Here's how the part is built. I have some questions about the finished solid (model axes, mm). Round coordinates to 2 decimals unless told otherwise and drop trailing zeros. Answer as a JSON object with one key per item and string values. Group by question number.
1) I want a section at A-A, the plane z = 3.25. Give the number of separate pieces and of enclosed holes in the cut face, then the cut area to 3 significant figures.
2) Will these pins go through, and if not, where does the flat tip stop? P1, Ø0.8, axis at y = 1, z = 16.5, coming from the -X side; P2, Ø3.5, axis at y = -41, z = 2, coming from the +X side; P3, Ø1.7, axis at y = 24.5, z = 16.5, coming from the +X side (3 decimals).
3) If I drill on line 1 along Y through (x, z) = (50, 5); line 2 along X through (y, z) = (56, 12.25) (1 decimal); line 3 along X through (y, z) = (-42, 1.75), over which ranges is the centre line in solid material (lowest first)? Write a range as [from, to].
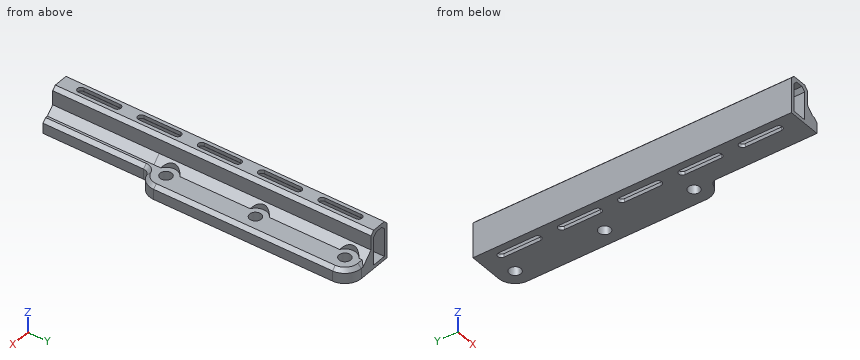
Autodesk Inventor part; units mm, degrees
ref_plane "Work Plane1" through (0, 0, 0) normal (0, 0, 1) x (1, 0, 0)
ref_plane "Work Plane2" through (40.2375, 90.7678, 31.75) normal (0, 0, 1) x (1, 0, 0)
ref_plane "Work Plane3" through (-55.775, -68.275, 0) normal (0, 0, 1) x (1, 0, 0)
ref_plane "Work Plane1" through (0, 0, 0) normal (0, 0, 1) x (1, 0, 0)
sketch "Sketch1" plane through (0, 0, 0) normal (0, 0, 1) x (1, 0, 0)
  circle A0 centre (50, -17.5) radius 2.6
  circle A1 centre (50, 22.5) radius 2.6
  circle A2 centre (50, 62.5) radius 2.6
  circle A3 centre (50, -17.5) radius 7.3625 construction
  circle A4 centre (50, 22.5) radius 7.3625 construction
  circle A5 centre (50, 62.5) radius 7.3625 construction
  line L0 (50, -24.8625) -> (42.6375, -24.8625)
  line L1 (42.6375, -24.8625) -> (42.6375, 69.8625)
  line L2 (42.6375, 69.8625) -> (50, 69.8625)
  line L3 (57.3625, -17.5) -> (57.3625, 62.5)
  arc A6 (50, -24.8625) -> (57.3625, -17.5) centre (50, -17.5) ccw
  arc A7 (57.3625, 62.5) -> (50, 69.8625) centre (50, 62.5) ccw
  circle A8 centre (50, -17.5) radius 5 construction
  point P0 (0, 0)
  dimension "d0" = 4.7625
  dimension "d1" = 10
extrude "Extrusion1" add sketch "Sketch1" along normal blind 6.175
sketch "Sketch2" plane through (0, 0, 6.175) normal (0, 0, 1) x (1, 0, 0)
  line L0 (42.6375, 69.8625) -> (42.6375, -24.8625)
  circle A0 centre (50, -17.5) radius 2.6
  circle A1 centre (50, -17.5) radius 5 construction
  line L1 (42.6375, -24.8625) -> (50, -24.8625) construction
  line L2 (44.225, -24.8625) -> (44.225, 69.8625)
  line L3 (42.6375, 69.8625) -> (44.225, 69.8625)
  line L4 (42.6375, -24.8625) -> (44.225, -24.8625)
  point P0 (0, 0)
  dimension "d4" = 10
  dimension "d34" = 1.5875
ref_plane "Work Plane2" through (40.2375, 90.7678, 31.75) normal (0, 0, 1) x (1, 0, 0)
extrude "Extrusion2" add sketch "Sketch2" along normal blind 9.525 contours L3 L2 L4 L0
chamfer "Chamfer1" distance 3.175 angle 45 1 edges at (44.225, 22.5, 6.175)
sketch "Sketch3" plane through (0, 0, 6.175) normal (0, 0, 1) x (1, 0, 0)
  circle A0 centre (50, -17.5) radius 2.6
  circle A1 centre (50, -17.5) radius 5
  circle A2 centre (50, 22.5) radius 2.6
  circle A3 centre (50, 62.5) radius 2.6
  circle A4 centre (50, 22.5) radius 5
  circle A5 centre (50, 62.5) radius 5
  point P0 (0, 0)
  point P1 (48.175, -15.6481)
  point P2 (48.175, -19.3519)
  point P3 (48.175, 24.3519)
  point P4 (48.175, 20.6481)
  point P5 (48.175, 64.3519)
  point P6 (48.175, 60.6481)
  dimension "d10" = 10
extrude "Extrusion3" cut sketch "Sketch3" along normal blind 25.4 contours A0 | A1 | A2 | A3 | A4 | A5
sketch "Sketch4" plane through (0, 0, 15.7) normal (0, 0, 1) x (1, 0, 0)
  line L0 (42.6375, -24.8625) -> (44.225, -24.8625)
  line L1 (44.225, -24.8625) -> (34.7, -24.8625)
  line L2 (34.7, -24.8625) -> (34.7, 69.8625)
  line L3 (34.7, 69.8625) -> (44.225, 69.8625)
  line L4 (44.225, 69.8625) -> (44.225, -24.8625)
  line L5 (44.225, 69.8625) -> (42.6375, 69.8625)
  line L6 (34.7, -24.8625) -> (36.2875, -24.8625)
  line L7 (36.2875, -24.8625) -> (36.2875, 69.8625)
  line L8 (36.2875, 69.8625) -> (34.7, 69.8625)
  line L9 (34.7, 69.8625) -> (34.7, -24.8625)
  line L10 (42.6375, 69.8625) -> (42.6375, -24.8625)
  point P0 (0, 0)
  dimension "d13" = 9.525
  dimension "d15" = 1.5875
  dimension "d16" = 1.5875
ref_plane "Work Plane3" through (-55.775, -68.275, 0) normal (0, 0, 1) x (1, 0, 0)
extrude "Extrusion4" add sketch "Sketch4" against normal up to surface (15.7 mm away) contours L1 L2 L3 L7
sketch "Sketch5" plane through (0, 0, 15.7) normal (0, 0, 1) x (1, 0, 0)
  line L0 (34.7, -24.8625) -> (34.7, 69.8625)
  line L1 (50, 69.8625) -> (42.6375, 69.8625)
  line L2 (34.7, -24.8625) -> (44.225, -24.8625)
  line L3 (44.225, -24.8625) -> (44.225, 69.8625)
  line L4 (44.225, 69.8625) -> (34.7, 69.8625)
  line L5 (34.7, 69.8625) -> (34.7, -24.8625)
  line L6 (44.225, -24.8625) -> (44.225, 69.8625)
  point P0 (0, 0)
extrude "Extrusion5" add sketch "Sketch5" along normal blind 1.5875
chamfer "Chamfer2" distance 1.5875 angle 45 4 edges at (44.225, 22.5, 17.2875) (34.7, 22.5, 17.2875) (36.2875, 22.5, 15.7) (42.6375, 22.5, 15.7)
sketch "Sketch7" plane through (42.6375, -24.8625, 0) normal (0, -1, 0) x (1, 0, 0)
  point P0 (-42.6375, 0)
sketch "Sketch8" plane through (42.6375, -24.8625, 0) normal (0, -1, 0) x (1, 0, 0)
  line L0 (-7.9375, 15.7) -> (-6.35, 17.2875)
  line L1 (-7.9375, 0) -> (-7.9375, 15.7)
  line L2 (-6.35, 0) -> (-7.9375, 0)
  line L3 (-6.35, 14.1125) -> (-6.35, 0)
  line L4 (-4.7625, 15.7) -> (-6.35, 14.1125)
  line L5 (-4.7625, 15.7) -> (-1.5875, 15.7)
  line L6 (0, 14.1125) -> (-1.5875, 15.7)
  line L7 (0, 0) -> (0, 14.1125)
  line L8 (0, 0) -> (7.3625, 0)
  line L9 (7.3625, 0) -> (7.3625, 6.175)
  line L10 (4.7625, 6.175) -> (7.3625, 6.175)
  line L11 (1.5875, 9.35) -> (4.7625, 6.175)
  line L12 (1.5875, 9.35) -> (1.5875, 15.7)
  line L13 (0, 17.2875) -> (1.5875, 15.7)
  line L14 (-6.35, 17.2875) -> (0, 17.2875)
  point P0 (-42.6375, 0)
ref_plane "Work Plane4" through (-290, -72.5, -10.037) normal (0, -1, 0) x (1, 0, 0)
extrude "Extrusion7" add sketch "Sketch8" along normal up to surface (47.6375 mm away)
fillet "Fillet1" radius 3.175 1 edges at (50, -24.8625, 3.0875)
sketch "Sketch9" plane through (0, 0, 17.2875) normal (0, 0, 1) x (1, 0, 0)
  line L0 (36.2875, 69.8625) -> (36.2875, -72.5)
  line L1 (42.6375, 69.8625) -> (42.6375, -72.5)
  line L2 (39.4625, -63.3595) -> (39.4625, -47.1256) construction
  line L3 (41.05, -63.3595) -> (41.05, -47.1256)
  line L4 (37.875, -47.1256) -> (37.875, -63.3595)
  arc A0 (37.875, -63.3595) -> (41.05, -63.3595) centre (39.4625, -63.3595) ccw
  arc A1 (41.05, -47.1256) -> (37.875, -47.1256) centre (39.4625, -47.1256) ccw
  line L5 (36.2875, -72.5) -> (42.6375, -72.5)
  line L6 (39.4625, -36.3976) -> (39.4625, -20.1637) construction
  line L7 (41.05, -36.3976) -> (41.05, -20.1637)
  line L8 (37.875, -20.1637) -> (37.875, -36.3976)
  arc A2 (37.875, -36.3976) -> (41.05, -36.3976) centre (39.4625, -36.3976) ccw
  arc A3 (41.05, -20.1637) -> (37.875, -20.1637) centre (39.4625, -20.1637) ccw
  line L9 (39.4625, -9.4357) -> (39.4625, 6.7982) construction
  line L10 (41.05, -9.4357) -> (41.05, 6.7982)
  line L11 (37.875, 6.7982) -> (37.875, -9.4357)
  arc A4 (37.875, -9.4357) -> (41.05, -9.4357) centre (39.4625, -9.4357) ccw
  arc A5 (41.05, 6.7982) -> (37.875, 6.7982) centre (39.4625, 6.7982) ccw
  line L12 (39.4625, 17.5262) -> (39.4625, 33.7601) construction
  line L13 (41.05, 17.5262) -> (41.05, 33.7601)
  line L14 (37.875, 33.7601) -> (37.875, 17.5262)
  arc A6 (37.875, 17.5262) -> (41.05, 17.5262) centre (39.4625, 17.5262) ccw
  arc A7 (41.05, 33.7601) -> (37.875, 33.7601) centre (39.4625, 33.7601) ccw
  line L15 (39.4625, 44.4881) -> (39.4625, 60.722) construction
  line L16 (41.05, 44.4881) -> (41.05, 60.722)
  line L17 (37.875, 60.722) -> (37.875, 44.4881)
  arc A8 (37.875, 44.4881) -> (41.05, 44.4881) centre (39.4625, 44.4881) ccw
  arc A9 (41.05, 60.722) -> (37.875, 60.722) centre (39.4625, 60.722) ccw
  line L18 (42.6375, 69.8625) -> (36.2875, 69.8625)
  point P0 (0, 0)
  point P1 (39.4625, -55.2425)
  point P2 (39.4625, -72.5)
  point P3 (39.4625, -64.947)
  point P4 (39.4625, -72.5)
  point P5 (39.4625, -28.2806)
  point P6 (39.4625, -1.3187)
  point P7 (39.4625, 25.6431)
  point P8 (39.4625, 52.605)
  point P9 (39.4625, 69.8625)
  point P10 (39.4625, 62.3095)
  point P11 (39.4625, -37.9851)
  point P12 (39.4625, -45.5381)
  point P13 (39.4625, -11.0232)
  point P14 (39.4625, -18.5762)
  point P15 (39.4625, 15.9387)
  point P16 (39.4625, 8.3857)
  point P17 (39.4625, 42.9006)
  point P18 (39.4625, 35.3476)
  dimension "d38" = 1.5875
  dimension "d39" = 7.553
  dimension "d40" = 16.2339
  dimension "d41" = 7.553
  dimension "d46" = 7.553
  dimension "d47" = 7.553
  dimension "d48" = 7.553
  dimension "d49" = 7.553
extrude "Extrusion8" cut sketch "Sketch9" against normal through all contours A0 L4 A1 L3 | A2 L8 A3 L7 | A4 L11 A5 L10 | A6 L14 A7 L13 | A8 L17 A9 L16
sketch "Sketch10" plane through (42.6375, 69.8625, 0) normal (0, 1, 0) x (1, 0, 0)
  line L0 (-6.35, -1.5875) -> (0, -1.5875)
  line L1 (-6.35, -14.1125) -> (-6.35, 0)
  line L2 (0, 0) -> (0, -14.1125)
  line L3 (26.1975, 0) -> (-54.11, 0)
  point P0 (-42.6375, 0)
  dimension "d53" = 1.5875
extrude "Extrusion9" add sketch "Sketch10" against normal up to surface (142.3625 mm away)
chamfer "Chamfer3" distance 1.5875 angle 45 5 edges at (50, -50.0239, 6.175) (55.9388, -21.8517, 6.175) (57.3625, 22.5, 6.175) (55.2061, 67.7061, 6.175) (48.6997, 69.8625, 6.175)
sketch "Sketch11" plane through (36.2875, -72.5, 1.5875) normal (0, 0, 1) x (1, 0, 0)
  line L0 (1.5875, 63.0643) -> (1.5875, 79.2982)
  arc A0 (4.7625, 79.2982) -> (1.5875, 79.2982) centre (3.175, 79.2982) ccw
  line L1 (4.7625, 79.2982) -> (4.7625, 63.0643)
  arc A1 (1.5875, 63.0643) -> (4.7625, 63.0643) centre (3.175, 63.0643) ccw
  line L2 (1.5875, 90.0262) -> (1.5875, 106.2601)
  arc A2 (4.7625, 106.2601) -> (1.5875, 106.2601) centre (3.175, 106.2601) ccw
  line L3 (4.7625, 106.2601) -> (4.7625, 90.0262)
  arc A3 (1.5875, 90.0262) -> (4.7625, 90.0262) centre (3.175, 90.0262) ccw
  line L4 (1.5875, 36.1024) -> (1.5875, 52.3363)
  arc A4 (4.7625, 52.3363) -> (1.5875, 52.3363) centre (3.175, 52.3363) ccw
  line L5 (4.7625, 52.3363) -> (4.7625, 36.1024)
  arc A5 (1.5875, 36.1024) -> (4.7625, 36.1024) centre (3.175, 36.1024) ccw
  line L6 (1.5875, 116.9881) -> (1.5875, 133.222)
  arc A6 (4.7625, 133.222) -> (1.5875, 133.222) centre (3.175, 133.222) ccw
  line L7 (4.7625, 133.222) -> (4.7625, 116.9881)
  arc A7 (1.5875, 116.9881) -> (4.7625, 116.9881) centre (3.175, 116.9881) ccw
  line L8 (1.5875, 9.1405) -> (1.5875, 25.3744)
  arc A8 (4.7625, 25.3744) -> (1.5875, 25.3744) centre (3.175, 25.3744) ccw
  line L9 (4.7625, 25.3744) -> (4.7625, 9.1405)
  arc A9 (1.5875, 9.1405) -> (4.7625, 9.1405) centre (3.175, 9.1405) ccw
  line L10 (0, 142.3625) -> (0, 0)
  line L11 (0, 0) -> (6.35, 0)
  line L12 (6.35, 142.3625) -> (6.35, 0)
  line L13 (6.35, 142.3625) -> (0, 142.3625)
  point P0 (-36.2875, 72.5)
extrude "Extrusion10" cut sketch "Sketch11" against normal blind 25.4 contours L0 A0 L1 A1 | L2 A2 L3 A3 | L4 A4 L5 A5 | L6 A6 L7 A7 | L8 A8 L9 A9
equation "\"d15\" = d16"
properties part number "CNC-028-WireTrack1" material "ABS Plastic"
Outcome:
{
 "1": {"separate pieces": "2", "enclosed holes": "3", "area": "1,890 mm^2"},
 "2": {"P1": "x = 35.1", "P2": "x = 50", "P3": "x = 44.225"},
 "3": {"line 1": "[-25.88, -20.1], [-14.9, 19.9], [25.1, 59.9], [65.1, 69.45]", "line 2": "[34.7, 36.3], [42.6, 44.2]", "line 3": "[34.7, 36.29], [42.64, 50]"}
}
